```python
from build123d import *

# Parameters (mm, degrees)
F0_R     = 5
F0_R_2   = 2.5
F1_DEPTH = 10
F2_DEPTH = 5
F3_SIZE  = 9.99999
F4_R     = 7
F5_R     = 10


# Not quite as in the source:
# - a fillet or chamfer is up to 0.001 mm smaller than in the source, because OpenCascade refuses the exact size


with BuildPart() as f1:
    # F0 (on Top) → F1 (new body)
    with BuildSketch(Plane.XY):
        Polygon((4.4427617314, -12.5), (20, -12.5), (20, 12.5), (4.4427617314, 12.5), (-4.4427617314, 12.5), (-20, 12.5), (-20, -12.5), (-4.4427617314, -12.5), align=None)
        with Locations((-10, 0)):
            Circle(F0_R, mode=Mode.SUBTRACT)
        with Locations((10, 0)):
            Circle(F0_R, mode=Mode.SUBTRACT)
        Polygon((-55.7045682747, -55.5137629639), (-4.4427617314, -12.5), (-20, -12.5), (-62.1324443715, -47.8533185328), align=None)
        Polygon((62.1324443715, -47.8533185328), (20, -12.5), (4.4427617314, -12.5), (55.7045682747, -55.5137629639), align=None)
        Polygon((4.4427617314, 12.5), (20, 12.5), (62.1324443715, 47.8533185328), (55.7045682747, 55.5137629639), align=None)
        Polygon((-20, 12.5), (-4.4427617314, 12.5), (-55.7045682747, 55.5137629639), (-62.1324443715, 47.8533185328), align=None)
        with Locations((10, 0)):
            Circle(F0_R)
        with Locations((10, 0)):
            Circle(F0_R_2, mode=Mode.SUBTRACT)
        with Locations((-10, 0)):
            Circle(F0_R)
        with Locations((-10, 0)):
            Circle(F0_R_2, mode=Mode.SUBTRACT)
    extrude(amount=F1_DEPTH)

    # F0 (on Top) → F2 (cut)
    with BuildSketch(Plane.XY):
        with Locations((-10, 0)):
            Circle(F0_R)
        with Locations((-10, 0)):
            Circle(F0_R_2, mode=Mode.SUBTRACT)
        with Locations((10, 0)):
            Circle(F0_R)
        with Locations((10, 0)):
            Circle(F0_R_2, mode=Mode.SUBTRACT)
    extrude(amount=F2_DEPTH, mode=Mode.SUBTRACT)

    # F3 (size 10 in the source; OpenCascade refuses exactly that, so slightly less here)
    f3_edges = [f1.edges().sort_by_distance(p)[0] for p in [
        (58.918506, -51.683541, 10),
        (58.918506, 51.683541, 10),
        (-58.918506, 51.683541, 10),
        (-58.918506, -51.683541, 10),
    ]]
    chamfer(f3_edges, length=F3_SIZE)

    # F4
    f4_edges = [f1.edges().sort_by_distance(p)[0] for p in [
        (4.442762, 12.5, 5),
        (-4.442762, 12.5, 5),
        (4.442762, -12.5, 5),
        (-4.442762, -12.5, 5),
        (-20, -12.5, 5),
        (-20, 12.5, 5),
        (20, -12.5, 5),
        (20, 12.5, 5),
    ]]
    fillet(f4_edges, radius=F4_R)

    # F5
    f5_edges = [f1.edges().sort_by_distance(p)[0] for p in [
        (-51.25807, 45.255671, 10),
        (-51.25807, -45.255671, 10),
        (51.25807, 45.255671, 10),
        (51.25807, -45.255671, 10),
    ]]
    fillet(f5_edges, radius=F5_R)


solid = f1.part
```
CAD build for the part. Positions are in the model's coordinates, mm. A direction names the side the tool comes from. Coordinates: 2 decimals unless noted, no trailing zeros. Loops run counter-clockwise (first coordinate to the right, second up) from the corner with the lowest first, then second, coordinate; pieces in that order, holes last. Notation, with made-up numbers: (13, 30.25) - (55, 30.25) arc R20 ccw to (55, 55.25) - close; hole circle Ø7 at (89, 46.25). An arc over 180 degrees is marked (long way). Return JSON: item names as keys, results as strings.
1. Band-saw the part on B-B (z = 2.5). Give the cut face in (x, y).
Result:
{"outline": "(-60.22, -46.25) - (-53.79, -53.91) - (-6.39, -14.14) arc R7 cw to (-1.89, -12.5) - (1.89, -12.5) arc R7 cw to (6.39, -14.14) - (53.79, -53.91) - (60.22, -46.25) - (22.5, -14.6) arc R7 cw to (20, -9.24) - (20, 9.24) arc R7 cw to (22.5, 14.6) - (60.22, 46.25) - (53.79, 53.91) - (6.39, 14.14) arc R7 cw to (1.89, 12.5) - (-1.89, 12.5) arc R7 cw to (-6.39, 14.14) - (-53.79, 53.91) - (-60.22, 46.25) - (-22.5, 14.6) arc R7 cw to (-20, 9.24) - (-20, -9.24) arc R7 cw to (-22.5, -14.6) - close; hole circle Ø10 at (-10, 0); hole circle Ø10 at (10, 0)"}
2. Probe L1, parallel to X at y = 35, z = 8.75; L2, parallel to Y at x = -10, z = 3.9; L3, parallel to X at y = -14, z = 5.75. List the from-to ranges inside material, lowest first. Write a range as from..to.
Result:
{"L1": "x = -46.81..-31.26, 31.26..46.81", "L2": "y = -17.16..-5, 5..17.16", "L3": "x = -21.87..-6.23, 6.23..21.87"}
3. Mould opens along Y. For faces 1 (the flat face through (0, 0, 0)), 2 (the flat face through (0, -12.5, 5)), 3 (the cylindrical face through (-20.674, 12.233, 5.07)), 4 (the cylindrical face through (-20.674, -12.233, 5.07)) say: released by +Y, released by -Y, zero draft, split by the parting line, or undercut.
Result:
{"face 1": "zero draft", "face 2": "released by -Y", "face 3": "undercut", "face 4": "undercut"}
4. Band-saw the part on A-A (y = 0). Give the cut face in (x, z).
Result:
{"outline": "(-20, 0) - (-15, 0) - (-15, 5) - (-12.5, 5) - (-12.5, 10) - (-20, 10) - close; (-7.5, 5) - (-5, 5) - (-5, 0) - (5, 0) - (5, 5) - (7.5, 5) - (7.5, 10) - (-7.5, 10) - close; (12.5, 5) - (15, 5) - (15, 0) - (20, 0) - (20, 10) - (12.5, 10) - close"}
5. 3-axis set-ups, long thin cutter, end or side, ignore diameter. For faces 5 (the flat face through (20, 0, 5)), 6 (the flat face through (-20, 0, 5)), 7 (the cylindrical face through (-4.26, -12.91, 5.07)): which of +Z, -Z, +X, -X, +Y, -Y reach the whole face in a straight line?
Result:
{"face 5": "+Z, -Z, +X", "face 6": "+Z, -Z, -X", "face 7": "+Z, -Z, -Y"}
6. Band-saw the part on D-D (y = -36). Give the cut face in (x, z), and give its area (3 significant figures).
Result:
{"outline": "(-48.01, 0) - (-32.45, 0) - (-32.45, 10) - (-48.01, 10) - close; (32.45, 0) - (48.01, 0) - (48.01, 10) - (32.45, 10) - close", "area": "311 mm2"}
7. Band-saw the part on C-C (x = 10). Give the cut face in (y, z).
Result:
{"outline": "(-17.16, 0) - (-5, 0) - (-5, 5) - (-2.5, 5) - (-2.5, 10) - (-17.16, 10) - close; (2.5, 5) - (5, 5) - (5, 0) - (17.16, 0) - (17.16, 10) - (2.5, 10) - close"}
8. Drop flat-ended pins along their axis: pin 1 (1 mm diameter, centred on x = -49.5, z = 4, fed in from -Y); pin 2 (6 mm diameter, centred on x = 10, y = 0, fed in from -Z); pin 3 (4 mm diameter, centred on x = -10, y = 0, fed in from -Z); pin 4 (6 mm diameter, centred on y = 7.5, z = 3, fed in from -X). Give the stop position or say it passes through.
Result:
{"pin 1": "stops at y = -50.73", "pin 2": "stops at z = 5", "pin 3": "passes through", "pin 4": "stops at x = -20.12"}
